```python
from build123d import *

# Parameters (mm, degrees)
F0_R      = 7.5
F0_R_2    = 2.65
F1_DEPTH  = 15
F2_R      = 11
F3_DEPTH  = 15
F4_DEPTH  = 15
F6_DEPTH  = 4.5
F7_SIZE   = 1
F9_DEPTH  = 25
F10_R     = 2.65
F11_DEPTH = 25


with BuildPart() as f1:
    # F0 (on Top) → F1 (new body)
    with BuildSketch(Plane.XY):
        Circle(F0_R)
        Circle(F0_R_2, mode=Mode.SUBTRACT)
    extrude(amount=F1_DEPTH)

    # F2 (on face) → F3 (join)
    with BuildSketch(Plane.XY.offset(15)):
        Circle(F2_R)
    extrude(amount=F3_DEPTH)

    # F2 (on face) → F4 (join)
    with BuildSketch(Plane.XY.offset(15)):
        Circle(F2_R)
    extrude(amount=F4_DEPTH)

    # F5 (on face) → F6 (cut)
    with BuildSketch(Plane.XY.offset(30)):
        Polygon((4, -2.309401), (4, 2.309401), (0, 4.618802), (-4, 2.309401), (-4, -2.309401), (0, -4.618802), align=None)
    extrude(amount=-F6_DEPTH, mode=Mode.SUBTRACT)

    # F7
    f7_edges = [f1.edges().sort_by_distance(p)[0] for p in [
        (-11, 0, 30),
        (-11, 0, 15),
    ]]
    chamfer(f7_edges, length=F7_SIZE)

    # F8 (on face) → F9 (cut)
    with BuildSketch(Plane.XY.offset(30)):
        Polygon((0, -10.23863), (-0.5, -10.98863), (0, -11.73863), (0.5, -10.98863), align=None)
        Polygon((1.957736, -10.824383), (2.612091, -11.444319), (2.932664, -10.601862), (2.27831, -9.981927), align=None)
        Polygon((4.317304, -10.117356), (5.093201, -10.576141), (5.218273, -9.683472), (4.442375, -9.224687), align=None)
        Polygon((6.460383, -8.903002), (7.318916, -9.177631), (7.242215, -8.279512), (6.383682, -8.004884), align=None)
        Polygon((8.279512, -7.242215), (9.177631, -7.318916), (8.903002, -6.460383), (8.004884, -6.383682), align=None)
        Polygon((9.683472, -5.218273), (10.576141, -5.093201), (10.117356, -4.317304), (9.224687, -4.442375), align=None)
        Polygon((10.601862, -2.932664), (11.444319, -2.612091), (10.824383, -1.957736), (9.981927, -2.27831), align=None)
        Polygon((10.98863, -0.5), (11.73863, 0), (10.98863, 0.5), (10.23863, 0), align=None)
        Polygon((10.824383, 1.957736), (11.444319, 2.612091), (10.601862, 2.932664), (9.981927, 2.27831), align=None)
        Polygon((10.117356, 4.317304), (10.576141, 5.093201), (9.683472, 5.218273), (9.224687, 4.442375), align=None)
        Polygon((8.903002, 6.460383), (9.177631, 7.318916), (8.279512, 7.242215), (8.004884, 6.383682), align=None)
        Polygon((7.242215, 8.279512), (7.318916, 9.177631), (6.460383, 8.903002), (6.383682, 8.004884), align=None)
        Polygon((5.218273, 9.683472), (5.093201, 10.576141), (4.317304, 10.117356), (4.442375, 9.224687), align=None)
        Polygon((2.932664, 10.601862), (2.612091, 11.444319), (1.957736, 10.824383), (2.27831, 9.981927), align=None)
        Polygon((0.5, 10.98863), (0, 11.73863), (-0.5, 10.98863), (0, 10.23863), align=None)
        Polygon((-1.957736, 10.824383), (-2.612091, 11.444319), (-2.932664, 10.601862), (-2.27831, 9.981927), align=None)
        Polygon((-4.317304, 10.117356), (-5.093201, 10.576141), (-5.218273, 9.683472), (-4.442375, 9.224687), align=None)
        Polygon((-6.460383, 8.903002), (-7.318916, 9.177631), (-7.242215, 8.279512), (-6.383682, 8.004884), align=None)
        Polygon((-8.279512, 7.242215), (-9.177631, 7.318916), (-8.903002, 6.460383), (-8.004884, 6.383682), align=None)
        Polygon((-9.683472, 5.218273), (-10.576141, 5.093201), (-10.117356, 4.317304), (-9.224687, 4.442375), align=None)
        Polygon((-10.601862, 2.932664), (-11.444319, 2.612091), (-10.824383, 1.957736), (-9.981927, 2.27831), align=None)
        Polygon((-10.98863, 0.5), (-11.73863, 0), (-10.98863, -0.5), (-10.23863, 0), align=None)
        Polygon((-10.824383, -1.957736), (-11.444319, -2.612091), (-10.601862, -2.932664), (-9.981927, -2.27831), align=None)
        Polygon((-10.117356, -4.317304), (-10.576141, -5.093201), (-9.683472, -5.218273), (-9.224687, -4.442375), align=None)
        Polygon((-8.903002, -6.460383), (-9.177631, -7.318916), (-8.279512, -7.242215), (-8.004884, -6.383682), align=None)
        Polygon((-7.242215, -8.279512), (-7.318916, -9.177631), (-6.460383, -8.903002), (-6.383682, -8.004884), align=None)
        Polygon((-5.218273, -9.683472), (-5.093201, -10.576141), (-4.317304, -10.117356), (-4.442375, -9.224687), align=None)
        Polygon((-2.932664, -10.601862), (-2.612091, -11.444319), (-1.957736, -10.824383), (-2.27831, -9.981927), align=None)
    extrude(amount=-F9_DEPTH, mode=Mode.SUBTRACT)

    # F10 (on face) → F11 (cut)
    with BuildSketch(Plane.XY.offset(25.5)):
        Circle(F10_R)
    extrude(amount=-F11_DEPTH, mode=Mode.SUBTRACT)


solid = f1.part
```
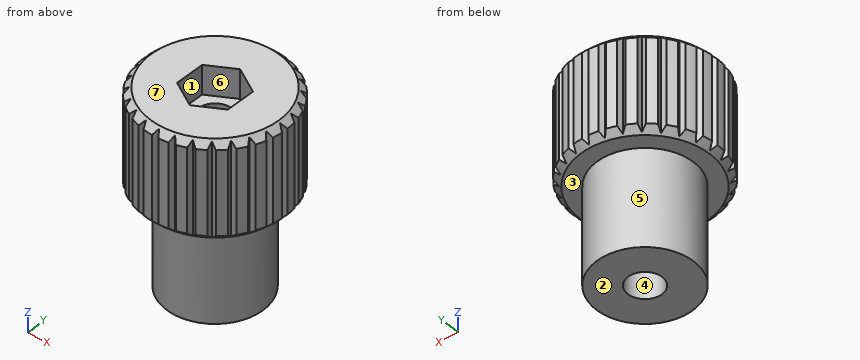
The listing builds one solid part. Answer for the finished solid, in the listing's coordinates (mm). Face numbers are marked on the shaded views. A direction names the side the tool comes from. Round coordinates to 2 decimals unless told otherwise and drop trailing zeros. Loops run counter-clockwise (first coordinate to the right, second up) from the corner with the lowest first, then second, coordinate; pieces in that order, holes last. Notation, with made-up numbers: (12, 40) - (69, 40) arc R15 ccw to (69, 55) - close; hole circle Ø11 at (-19.75, 8). An arc over 180 degrees is marked (long way). Return JSON: item names as keys, results as strings. Group by question number.
1. Which of the six approach directions +Z, -Z, +X, -X, +Y, -Y give full straight-line access (tool end or side, diameter ignored) to the marked faces 1, 2 and 3?
2. Consider probe 1 along Y at (x, z) = (0, 11); probe 2 along Z at (x, y) = (-3.25, 8.5); probe 3 along X at (y, z) = (-1.75, 5.25). Determine where each line is inside the solid, lowest interval first.
3. The part is cut by section A-A on z = 13.75. Determine the outline of the cut face in (x, y), then the cut area to 3 significant figures.
4. The mould has two halves that part along Y. Classify the marked faces 4, 5, 6 and 7: pulls with the +Y half, pulls with the -Y half, needs draft (parallel to the pull), parting line crosses it, or undercut.
5. Each of these flat-tipped pins is pushed along its axis until it touches: P1, Ø2, axis at x = 2, z = 15.5, coming from the +Y side; P2, Ø5, axis at x = -8, z = 21, coming from the -Y side; P3, Ø10, axis at x = -2.5, y = -0.5, coming from the -Z side; P4, Ø8, axis at y = 6.5, z = 16, coming from the +X side. Where does it stop, or does it pass through?
Resolved:
{
 "1": {"face 1": "+Z", "face 2": "-Z, +X, -X, +Y, -Y", "face 3": "-Z"},
 "2": {"probe 1": "y = -7.5 to -2.65, 2.65 to 7.5", "probe 2": "z = 15 to 30", "probe 3": "x = -7.29 to -1.99, 1.99 to 7.29"},
 "3": {"outline": "circle Ø15 at (0, 0); hole circle Ø5.3 at (0, 0)", "area": "155 mm²"},
 "4": {"face 4": "undercut", "face 5": "parting line crosses it", "face 6": "undercut", "face 7": "needs draft"},
 "5": {"P1": "stops at y = 10.94", "P2": "stops at y = -9.53", "P3": "stops at z = 0", "P4": "stops at x = 10.6"}
}
